```python
from build123d import *

# Parameters (mm, degrees)
BOSS_EXTRUDE1_DEPTH = 20
SKETCH2_R           = 4
CUT_EXTRUDE2_DEPTH  = 8
CUT_EXTRUDE4_DEPTH  = 10
SKETCH4_R           = 2.6
CUT_EXTRUDE5_DEPTH  = 1.5
SKETCH6_W           = 2.5
SKETCH6_H           = 20
SKETCH6_W_2         = 10
BOSS_EXTRUDE3_DEPTH = 5


with BuildPart() as part:
    # Sketch1 → Boss-Extrude1 (new body)
    with BuildSketch(Plane(origin=(0, 0, 0), x_dir=(1, 0, 0), z_dir=(0, 1, 0))):
        with BuildLine():
            Line((-30.801242739, -7.293134051), (-30.801242739, 22.74889672))
            ThreePointArc((-30.801242739, 22.74889672), (-52.993630894, 31.941284876), (-43.801242739, 9.74889672))
            Line((-43.801242739, 9.74889672), (-43.801242739, -37.25110328))
            Line((-43.801242739, -37.25110328), (-41.301242739, -37.25110328))
            Line((-41.301242739, -37.25110328), (-41.301242739, 22.74889672))
            Line((-41.301242739, 22.74889672), (-43.801242739, 22.74889672))
            Line((-43.801242739, 22.74889672), (-43.801242739, 12.24889672))
            ThreePointArc((-43.801242739, 12.24889672), (-51.225863941, 30.173517923), (-33.301242739, 22.74889672))
            Line((-33.301242739, 22.74889672), (-33.301242739, -37.25110328))
            Line((-33.301242739, -37.25110328), (-23.301242739, -37.25110328))
            Line((-23.301242739, -37.25110328), (-23.301242739, -7.25110328))
            Line((-23.301242739, -7.25110328), (-30.801242739, -7.293134051))
        make_face()
    extrude(amount=BOSS_EXTRUDE1_DEPTH)

    # Sketch2 → Cut-Extrude2 (cut)
    with BuildSketch(Plane.ZY.offset(33.301242739)):
        with Locations((17.25110328, 10)):
            Circle(SKETCH2_R)
        with Locations((32.25110328, 10)):
            Circle(SKETCH2_R)
    extrude(amount=-CUT_EXTRUDE2_DEPTH, mode=Mode.SUBTRACT)

    # Sketch3 → Cut-Extrude4 (cut)
    with BuildSketch(Plane(origin=(-23.301242739, 0, 0), x_dir=(0, 0, -1), z_dir=(1, 0, 0))):
        Polygon((-24.75110328, 10), (-27.75110328, 10.5), (-27.75110328, 9.5), align=None)
        Polygon((-21.75110328, 10.5), (-27.75110328, 10.5), (-24.75110328, 10), align=None)
        Polygon((-21.75110328, 10.5), (-24.75110328, 10), (-21.75110328, 9.5), align=None)
        Polygon((-21.75110328, 9.5), (-24.75110328, 10), (-27.75110328, 9.5), align=None)
        Polygon((-17.25110328, 10), (-20.25110328, 10.5), (-20.25110328, 9.5), align=None)
        Polygon((-14.25110328, 10.5), (-17.25110328, 10), (-14.25110328, 9.5), align=None)
        Polygon((-14.25110328, 10.5), (-20.25110328, 10.5), (-17.25110328, 10), align=None)
        Polygon((-14.25110328, 9.5), (-17.25110328, 10), (-20.25110328, 9.5), align=None)
        Polygon((-29.25110328, 10.5), (-32.25110328, 10), (-29.25110328, 9.5), align=None)
        Polygon((-29.25110328, 10.5), (-35.25110328, 10.5), (-32.25110328, 10), align=None)
        Polygon((-32.25110328, 10), (-35.25110328, 10.5), (-35.25110328, 9.5), align=None)
        Polygon((-29.25110328, 9.5), (-32.25110328, 10), (-35.25110328, 9.5), align=None)
    extrude(amount=-CUT_EXTRUDE4_DEPTH, mode=Mode.SUBTRACT)

    # Sketch4 → Cut-Extrude5 (cut)
    with BuildSketch(Plane.ZY.offset(33.301242739)):
        with Locations((24.75110328, 10)):
            Circle(SKETCH4_R)
    extrude(amount=-CUT_EXTRUDE5_DEPTH, mode=Mode.SUBTRACT)

    # Sketch6 → Boss-Extrude3 (add)
    with BuildSketch(Plane.XY.offset(37.25110328)):
        with Locations((-42.551242739, 10)):
            Rectangle(SKETCH6_W, SKETCH6_H)
        with Locations((-28.301242739, 10)):
            Rectangle(SKETCH6_W_2, SKETCH6_H)
    extrude(amount=BOSS_EXTRUDE3_DEPTH)


solid = part.part
```
CAD build for the part. Positions are in the model's coordinates, mm. A direction names the side the tool comes from. Coordinates: 2 decimals unless noted, no trailing zeros. Order: outer loops, then holes, each group sorted by start corner. A loop starts at its lowest first (then second) coordinate and runs counter-clockwise, first axis right, second up. Notation, with made-up numbers: (32.25, 19.25) - (42.25, 19.25) arc R28 ccw to (42.25, 45.25) - close; hole circle Ø3 at (41.25, 30). An arc over 180 degrees is marked (long way). Use a Markdown table: item, result. Add a question column.
(1) Saw through at D-D (z = 34.5). Give the cut face in (x, y), then the cut area to 3 significant figures.
(2) Drill centre lines: line 1 along Y through (x, z) = (-28.5, 22); line 2 along X through (y, z) = (10.25, -6.5); line 3 along X through (y, z) = (18.75, -18.5). Where is each one in solid material? Low to high. Write a range as [from, to].
(3) Saw through at B-B (x = -52.5). Give the cut face in (y, z), then the cut area to 3 significant figures.
(4) Saw through at C-C (y = 2.25). Give the cut face in (x, z), then the cut area to 3 significant figures.
(5) Pull direction Z, two halves, no side cores. Call faces 4 (the face through (-52.685, 9.86, -32.239)), 5 (the face through (-41.301, 10, 9)), 6 (the face through (-28, 10.5, 25)): +Z half, -Z half, draft (parallel to the pull), parting line (faces both ways), or undercut.
(6) Which spindle directions (+Z, -Z, +X, -X, +Y, -Y) get a long thin tool onto all of the face, cutting with end or side? Do faces 1 (the face through (-43.801, 10, 16)), 2 (the face through (-24, 10.5, 32)), 3 (the face through (-25.301, 9, 17)). Say none if no direction does.
(7) Saw through at A-A (z = 2). Give the cut face in (x, y), then the cut area to 3 significant figures.
(8) Flat gauge pins, fed straight in: pin 1 (6 mm diameter, centred on x = -26.5, z = -11.5, fed in from -Y); pin 2 (4 mm diameter, centred on y = 10, z = 19, fed in from -X); pin 3 (1 mm diameter, centred on y = 5.5, z = -18, fed in from -X); pin 4 (2 mm diameter, centred on x = -37, y = 15.5, fed in from -Z). Where does each tip first touch, or does it go through?
Solved:
| question | item | result |
|---|---|---|
| 1 | outline | (-43.8, 0) - (-41.3, 0) - (-41.3, 20) - (-43.8, 20) - close; (-33.3, 0) - (-23.3, 0) - (-23.3, 9.5) - (-25.3, 9.5) - (-25.3, 6.69) - (-33.3, 6.69) - close; (-33.3, 13.31) - (-25.3, 13.31) - (-25.3, 10.5) - (-23.3, 10.5) - (-23.3, 20) - (-33.3, 20) - close |
| 1 | area | 195 mm² |
| 2 | line 1 | y = [0, 9.5], [10.5, 20] |
| 2 | line 2 | x = [-43.8, -41.3], [-33.3, -30.8] |
| 2 | line 3 | x = [-56.09, -53.4], [-43.8, -41.3], [-33.3, -30.8] |
| 3 | outline | (0, -32.41) - (20, -32.41) - (20, -28.63) - (0, -28.63) - close; (0, -16.87) - (20, -16.87) - (20, -13.09) - (0, -13.09) - close |
| 3 | area | 151 mm² |
| 4 | outline | (-43.8, -22.75) - (-41.3, -22.75) - (-41.3, 42.25) - (-43.8, 42.25) - (-43.8, -9.75) arc R13 ccw (long way) to (-30.8, -22.75) - (-30.8, 7.29) - (-23.3, 7.25) - (-23.3, 42.25) - (-33.3, 42.25) - (-33.3, -22.75) arc R10.5 cw (long way) to (-43.8, -12.25) - close |
| 4 | area | 726 mm² |
| 5 | face 4 | parting line |
| 5 | face 5 | draft |
| 5 | face 6 | undercut |
| 6 | face 1 | +Z, -X, +Y, -Y |
| 6 | face 2 | +X |
| 6 | face 3 | none |
| 7 | outline | (-43.8, 0) - (-41.3, 0) - (-41.3, 20) - (-43.8, 20) - close; (-33.3, 0) - (-30.8, 0) - (-30.8, 20) - (-33.3, 20) - close |
| 7 | area | 100 mm² |
| 8 | pin 1 | passes through |
| 8 | pin 2 | stops at x = -43.8 |
| 8 | pin 3 | stops at x = -56.09 |
| 8 | pin 4 | stops at z = -34.38 |
